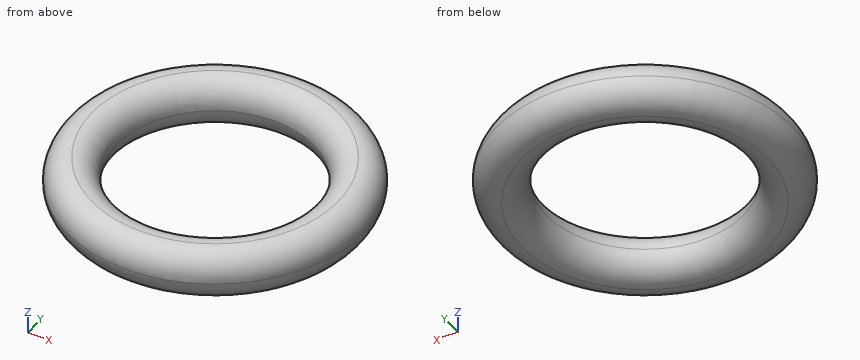
from build123d import *

# Parameters (mm, degrees)
SKETCH1_R           = 76.2
SKETCH1_R_2         = 50.8
BOSS_EXTRUDE1_DEPTH = 25.4
FILLET1_R           = 12.7
FILLET2_R           = 12.7


with BuildPart() as part:
    # Sketch1 → Boss-Extrude1 (new body)
    with BuildSketch(Plane.XY):
        Circle(SKETCH1_R)
        Circle(SKETCH1_R_2, mode=Mode.SUBTRACT)
    extrude(amount=BOSS_EXTRUDE1_DEPTH)

    # Fillet1
    fillet1_edges = [part.edges().sort_by_distance(p)[0] for p in [
        (-76.2, 0, 0),
        (-76.2, 0, 25.4),
    ]]
    fillet(fillet1_edges, radius=FILLET1_R - 0.0001)  # a hair under: the kernel refuses the full size

    # Fillet2
    fillet2_edges = [part.edges().sort_by_distance(p)[0] for p in [
        (-50.8, 0, 0),
        (-50.8, 0, 25.4),
    ]]
    fillet(fillet2_edges, radius=FILLET2_R - 0.0001)  # a hair under: the kernel refuses the full size


solid = part.part
Model file for the job. Use its own axes, mm. Give positions to 0.01 mm unless a question says otherwise; leave off trailing zeros. Order: outer loops, then holes, each group sorted by start corner. A loop starts at its lowest first (then second) coordinate and runs counter-clockwise, first axis right, second up. Notation, with made-up numbers: (-36, -38) - (13, -38) arc R18 cw to (13, -10) - close; hole circle Ø6 at (28, 14). An arc over 180 degrees is marked (long way). One line per item, written item: value.
Item 1: Slice it at D-D (z = 2.5). List the corners of the cut face in (x, y).
Response values:
outline: circle Ø142.13 at (0, 0); hole circle Ø111.87 at (0, 0)
Item 2: Wall check: line 1 (Y direction, x = 0, z = 12.7); line 2 (X direction, y = 7, z = 22.25); line 3 (Y direction, x = 26, z = 2). Give the ranges that are in metal, low to high.
Response values:
line 1: -76.2 to -50.8, 50.8 to 76.2
line 2: -71.53 to -54.68, 54.68 to 71.53
line 3: -65.36 to -50.34, 50.34 to 65.36
Item 3: Slice it at C-C (z = 16.75). List the corners of the cut face in (x, y).
Response values:
outline: circle Ø151.07 at (0, 0); hole circle Ø102.93 at (0, 0)
Item 4: Pin check, flat tips, straight feed: pin 1 Ø1 at (x, z) = (-13.5, 11) entering from +Y; pin 2 Ø4 at (y, z) = (28, 11) entering from -X; pin 3 Ø10 at (x, z) = (19, 18) entering from +Y. Stop position of each tip, or through.
Response values:
pin 1: y = 74.99
pin 2: x = -71.54
pin 3: y = 74.5
